Design review of the part built by this model. Coordinates are the model's own, in mm. Coordinates: 2 decimals unless noted, no trailing zeros. Loops run counter-clockwise (first coordinate to the right, second up) from the corner with the lowest first, then second, coordinate; pieces in that order, holes last. Notation, with made-up numbers: M 2.25,14 L 55.25,14 A31 ccw 55.25,43 Z; hole C 22.5,-15.75 d6. An arc over 180 degrees is marked long. One line per item, written item: value.
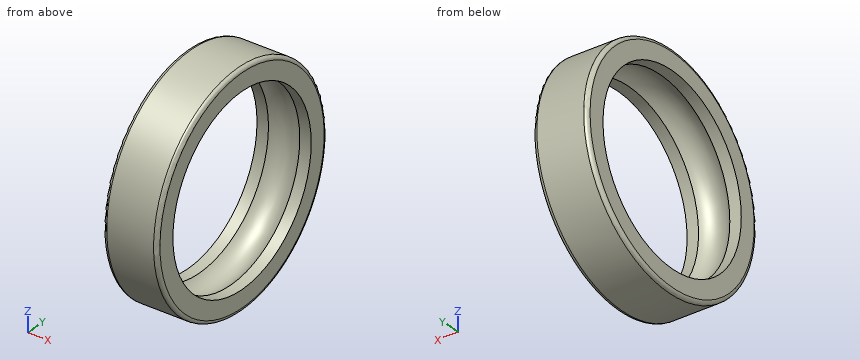
```python
from build123d import *

# Parameters (mm, degrees)
FILLET1_R    = 2.1
SCALE1_SCALE = 0.35


with BuildPart() as part:
    # Sketch1 → Revolve1 (revolve)
    with BuildSketch(Plane.XY, mode=Mode.PRIVATE) as revolve1_sk:
        with BuildLine():
            Line((-15.5, 65), (15.5, 65))
            Line((15.5, 65), (15.5, 53))
            Line((15.5, 53), (8.94427191, 53))
            ThreePointArc((8.94427191, 53), (0, 57), (-8.94427191, 53))
            Line((-8.94427191, 53), (-15.5, 53))
            Line((-15.5, 53), (-15.5, 65))
        make_face()
    revolve(revolve1_sk.sketch.rotate(Axis((-25.358454362, 0, 0), (1, 0, 0)), 90), axis=Axis((-25.358454362, 0, 0), (1, 0, 0)))

    # Fillet1
    fillet1_edges = [part.edges().sort_by_distance(p)[0] for p in [
        (15.5, 0, -65),
        (-15.5, 0, -65),
    ]]
    fillet(fillet1_edges, radius=FILLET1_R)


with BuildPart() as part_1:
    # Scale1: scaled about (0, 0, 0)
    add(part.part.scale(SCALE1_SCALE))


solid = part_1.part
```
(1) Insertion check: pin 1 (2 mm diameter, centred on x = 0, y = 17, fed in from -Z); pin 2 (1 mm diameter, centred on x = -2.5, z = 13.5, fed in from -Y); pin 3 (1.5 mm diameter, centred on x = 2.5, z = -12, fed in from -Y); pin 4 (5 mm diameter, centred on x = 2, y = -2.5, fed in from -Z). Each pin has a flat end and moves straight along its axis. Give the tip position at first contact, or say it passes through.
Reply:
pin 1: stops at z = -16.17
pin 2: stops at y = -18.67
pin 3: stops at y = -19.77
pin 4: stops at z = -22.75
(2) We need section C-C on x = -4. State the section outline as (y, z) points, then the cut area to 3 significant figures.
Reply:
outline: C 0,0 d45.5; hole C 0,0 d37.1
area: 545 mm2
(3) We need section D-D on x = 1.75. State the section outline as (y, z) points.
Reply:
outline: C 0,0 d45.5; hole C 0,0 d39.14
(4) To check wall thickness, follow line 1 along Y through (x, z) = (-4.1, 0); line 2 along Z through (x, y) = (3, 3); line 3 along Z through (x, y) = (4, 12.5). State the ranges of each line that lie inside material, in increasing order. Write a range as [from, to].
Reply:
line 1: y = [-22.75, -18.55], [18.55, 22.75]
line 2: z = [-22.55, -18.45], [18.45, 22.55]
line 3: z = [-19.01, -13.71], [13.71, 19.01]
